Autodesk Inventor part; units mm, degrees
ref_plane "Combination_Module_XY" through (0, 0, 0) normal (1, 0, 0) x (0, 0, -1)
ref_plane "Combination_Module_YZ" through (0, 0, 0) normal (0, 0, -1) x (0, 1, 0)
ref_plane "Combination_Module_ZX" through (0, 0, 0) normal (0, 1, 0) x (1, 0, 0)
sketch "Sketch_1" plane through (0, 0, 0) normal (0, 0, 1) x (1, 0, 0)
  line L0 (29, 0) -> (0, 0)
  line L1 (0, 5.3) -> (0.7, 5.3)
  line L2 (0.7, 5.3) -> (0.7, 5.6)
  line L3 (0.7, 5.6) -> (1.05, 5.6)
  line L4 (1.05, 5.6) -> (1.05, 5)
  line L5 (1.05, 5) -> (27.95, 5)
  line L6 (27.95, 5) -> (27.95, 5.6)
  line L7 (27.95, 5.6) -> (28.3, 5.6)
  line L8 (28.3, 5.6) -> (28.3, 5.3)
  line L9 (28.3, 5.3) -> (29, 5.3)
  line L10 (29, 5.3) -> (29, 8.9)
  arc A0 (29, 8.9) -> (28.4, 9.5) centre (28.4, 8.9) ccw
  line L11 (28.4, 9.5) -> (6, 9.5)
  line L12 (6, 9.5) -> (6, 19.7)
  line L13 (6, 19.7) -> (5.7, 20)
  line L14 (5.7, 20) -> (0.3, 20)
  line L15 (0.3, 20) -> (0, 19.7)
  line L16 (0, 19.7) -> (0, 5.3)
revolve "Revolution1" add sketch "Sketch_1" angle 360 about axis through (29, 0, 0) along (1, 0, 0)
sketch "Sketch_2" plane through (0, 0, 0) normal (1, 0, 0) x (0, 1, 0)
  line L0 (-30, 30) -> (-30, -30)
  line L1 (-30, -30) -> (30, -30)
  line L2 (30, -30) -> (30, 30)
  line L3 (30, 30) -> (-30, 30)
  line L4 (-1.2132, 20) -> (-20, 1.2132)
  line L5 (-20, 1.2132) -> (-20, -1.2132)
  line L6 (-20, -1.2132) -> (-1.2132, -20)
  line L7 (-1.2132, -20) -> (1.2132, -20)
  line L8 (1.2132, -20) -> (20, -1.2132)
  line L9 (20, -1.2132) -> (20, 1.2132)
  line L10 (20, 1.2132) -> (1.2132, 20)
  line L11 (1.2132, 20) -> (-1.2132, 20)
extrude "Extrusion1" cut sketch "Sketch_2" along normal blind 6
sketch "Sketch3" plane through (0, 0, 0) normal (-1, 0, 0) x (0, 0, 1)
  point P0 (0, 14.5)
hole "Hole1" at (0, 14.5, 0) direction (1, 0, 0) diameter 4.5 depth 6 counterbore diameter 7.5 counterbore depth 4.1
sketch "Sketch4" plane through (0, 0, 0) normal (-1, 0, 0) x (0, 0, 1)
  point P0 (0, -14.5)
hole "Hole2" at (0, -14.5, 0) direction (1, 0, 0) diameter 4.5 depth 6 counterbore diameter 7.5 counterbore depth 4.1
sketch "Sketch5" plane through (0, 0, 0) normal (-1, 0, 0) x (0, 0, 1)
  point P0 (-14.5, 0)
hole "Hole3" at (0, 0, -14.5) direction (1, 0, 0) diameter 4.5 depth 6 counterbore diameter 7.5 counterbore depth 4.1
sketch "Sketch6" plane through (0, 0, 0) normal (-1, 0, 0) x (0, 0, 1)
  point P0 (14.5, 0)
hole "Hole4" at (0, 0, 14.5) direction (1, 0, 0) diameter 4.5 depth 6 counterbore diameter 7.5 counterbore depth 4.1
ref_plane "Combination_Module_XY" through (0, 0, 0) normal (1, 0, 0) x (0, 0, -1)
ref_plane "Combination_Module_YZ" through (0, 0, 0) normal (0, 0, -1) x (0, 1, 0)
ref_plane "Combination_Module_ZX" through (0, 0, 0) normal (0, 1, 0) x (1, 0, 0)
properties part number "C-LHFS10"
Input: part model. Units: mm. Frame: model coordinates. A direction names the side the tool comes from. Round coordinates to 2 decimals unless told otherwise and drop trailing zeros. Loops run counter-clockwise (first coordinate to the right, second up) from the corner with the lowest first, then second, coordinate; pieces in that order, holes last. Notation, with made-up numbers: M -11,84.25 L 28,84.25 A18 cw 28,106.25 Z; hole C 26.5,33 d10. An arc over 180 degrees is marked long. Answer in a Markdown table with one row per item. Add a question column.
1. Mould query, pull axis Z, two halves, no side actions, for faces 1 (the face through (3, 0, -20)), 2 (the face through (6, -9, -4)), 3 (the face through (2.08, -10.84, -0.81)), 4 (the face through (4.1, 16, 2)). Classes: released by +Z, released by -Z, zero draft, split by the parting line, or undercut.
2. Section C-C (x = 14.25). Output: boundary loops of the cut face in (y, z), and give its area (3 significant figures).
3. Ray query, probe 1 along Z at (x, y) = (2.25, 0); probe 2 along Z at (x, y) = (5, 0); probe 3 along X at (y, z) = (-6, 12.5). Return the intervals inside material, ascending.
4. Contact query for flat-ended pins moving along their axis: pin 1 (10 mm diameter, centred on x = 26, z = 4.5, fed in from -Y); pin 2 (2.5 mm diameter, centred on y = 0, z = -14.5, fed in from -X); pin 3 (6 mm diameter, centred on y = 0, z = 14.5, fed in from -X); pin 4 (1.5 mm diameter, centred on x = 24.5, z = 2, fed in from -Y). Output: stop coordinate, or through.
5. Set-up query: faces 5 (the face through (29, 4, -4)), 6 (the face through (4.1, -13, 2)), 7 (the face through (0, 0, 6)), 8 (the face through (28.655, 4.896, -2.03)), 9 (the face through (0.877, -5.595, 0.246)). Return all of +Z, -Z, +X, -X, +Y, -Y with unobstructed straight access to the full face (end or side cutting, diameter ignored); none if empty.
6. Section A-A (y = -13). Output: boundary loops of the cut face in (x, z).
7. Section B-B (z = 16). Output: boundary loops of the cut face in (x, y).
8. Section D-D (y = 0). Give the number of separate pieces and of enclosed holes in the cut face, and give its area (3 significant figures).
Values follow:
| question | item | result |
|---|---|---|
| 1 | face 1 | released by -Z |
| 1 | face 2 | zero draft |
| 1 | face 3 | undercut |
| 1 | face 4 | undercut |
| 2 | outline | C 0,0 d19; hole C 0,0 d10 |
| 2 | area | 205 mm^2 |
| 3 | probe 1 | -20 to -18.25, -10.75 to -5, 5 to 10.75, 18.25 to 20 |
| 3 | probe 2 | -20 to -16.75, -12.25 to -5, 5 to 12.25, 16.75 to 20 |
| 3 | probe 3 | 0 to 6 |
| 4 | pin 1 | y = -9.5 |
| 4 | pin 2 | through |
| 4 | pin 3 | x = 4.1 |
| 4 | pin 4 | y = -9.42 |
| 5 | face 5 | +Z, -Z, +X, +Y, -Y |
| 5 | face 6 | -X |
| 5 | face 7 | +Z, -Z, -X, +Y, -Y |
| 5 | face 8 | +X |
| 5 | face 9 | none |
| 6 | outline | M 0,-8.21 L 6,-8.21 L 6,-1.68 L 4.1,-1.68 L 4.1,-3.44 L 0,-3.44 Z; M 0,3.44 L 4.1,3.44 L 4.1,1.68 L 6,1.68 L 6,8.21 L 0,8.21 Z |
| 7 | outline | M 0,-5.21 L 6,-5.21 L 6,-1.68 L 4.1,-1.68 L 4.1,-3.44 L 0,-3.44 Z; M 0,3.44 L 4.1,3.44 L 4.1,1.68 L 6,1.68 L 6,5.21 L 0,5.21 Z |
| 8 | separate pieces | 4 |
| 8 | enclosed holes | 0 |
| 8 | area | 306 mm^2 |
